The listing builds one solid part. Answer for the finished solid, in the listing's coordinates (mm). Coordinates: 2 decimals unless noted, no trailing zeros. Write each loop counter-clockwise with the first axis right and the second up, starting at its lowest first coordinate (ties: lowest second). Pieces come first, ordered by that corner, then holes. Notation, with made-up numbers: M 71.5,20.5 L 79.5,20.5 A18 ccw 79.5,41.5 Z; hole C 69,28 d5. An arc over 180 degrees is marked long. Answer as CSV lines item,"result".
```python
from build123d import *

# Parameters (mm, degrees)
F0_W     = 43
F0_H     = 80
F0_R     = 3
F0_W_2   = 36
F0_H_2   = 52.5
F1_DEPTH = 0.8


with BuildPart() as f1:
    # F0 (on Top) → F1 (new body)
    with BuildSketch(Plane.XY):
        with Locations((2.4, -3.5)):
            Rectangle(F0_W, F0_H)
        with Locations((-13.1, -38.5)):
            Circle(F0_R, mode=Mode.SUBTRACT)
        with Locations((17.9, -38.5)):
            Circle(F0_R, mode=Mode.SUBTRACT)
        with Locations((-13.1, 31.5)):
            Circle(F0_R, mode=Mode.SUBTRACT)
        with Locations((2.4, -3.5)):
            Rectangle(F0_W_2, F0_H_2, mode=Mode.SUBTRACT)
        with Locations((17.9, 31.5)):
            Circle(F0_R, mode=Mode.SUBTRACT)
    extrude(amount=F1_DEPTH)


solid = f1.part
```
Q1. Find section D-D (y = 31.5). Give the vertices of the cut face in (x, z), and give its area (3 significant figures).
Output:
outline,"M -19.1,0 L -16.1,0 L -16.1,0.8 L -19.1,0.8 Z; M -10.1,0 L 14.9,0 L 14.9,0.8 L -10.1,0.8 Z; M 20.9,0 L 23.9,0 L 23.9,0.8 L 20.9,0.8 Z"
area,"24.8 mm2"
Q2. Straight lines are drawn through the part: line 1 (Y direction, x = 17.9, z = 0.2); line 2 (X direction, y = 17.5, z = 0.45); line 3 (X direction, y = -37.5, z = 0.5). For each, find the intervals that lie inside material, in ascending order.
Output:
line 1,"-43.5 to -41.5, -35.5 to -29.75, 22.75 to 28.5, 34.5 to 36.5"
line 2,"-19.1 to -15.6, 20.4 to 23.9"
line 3,"-19.1 to -15.93, -10.27 to 15.07, 20.73 to 23.9"
Q3. A flat-ended cylindrical pin translates along its axis: pin 1 Ø2 at (x, y) = (19, -12.5) entering from +Z. Find the tip coordinate at first contact, or state that the pin passes through.
Output:
pin 1,"through"
Q4. Find section A-A (y = -18). Give the vertices of the cut face in (x, z), and give its area (3 significant figures).
Output:
outline,"M -19.1,0 L -15.6,0 L -15.6,0.8 L -19.1,0.8 Z; M 20.4,0 L 23.9,0 L 23.9,0.8 L 20.4,0.8 Z"
area,"5.60 mm2"
Q5. Find section C-C (z = 0.55). Give the vertices of the cut face in (x, y), and give its area (3 significant figures).
Output:
outline,"M -19.1,-43.5 L 23.9,-43.5 L 23.9,36.5 L -19.1,36.5 Z; hole C -13.1,-38.5 d6; hole C -13.1,31.5 d6; hole M -15.6,-29.75 L 20.4,-29.75 L 20.4,22.75 L -15.6,22.75 Z; hole C 17.9,-38.5 d6; hole C 17.9,31.5 d6"
area,"1,440 mm2"
Q6. The mould has two halves that part along X. Classify faces 1 (the cylindrical face through (15.69, 33.53, 0.39)), 2 (the flat face through (21, 6, 0.8)): pulls with the +X half, pulls with the -X half, needs draft (parallel to the pull), parting line crosses it, or undercut.
Output:
face 1,"undercut"
face 2,"needs draft"
Q7. Find section B-B (x = 1.5). Give the vertices of the cut face in (y, z).
Output:
outline,"M -43.5,0 L -29.75,0 L -29.75,0.8 L -43.5,0.8 Z; M 22.75,0 L 36.5,0 L 36.5,0.8 L 22.75,0.8 Z"
